```python
from build123d import *

# Parameters (mm, degrees)
EXTRUDE_2_DEPTH     = 10
SKETCH_2_R          = 10
CUT_EXTRUDE_1_DEPTH = 10
SKETCH_3_R          = 10
CUT_EXTRUDE_2_DEPTH = 10


with BuildPart() as part:
    # Эскиз1 → Бобышка-Вытянуть2 (new body)
    with BuildSketch(Plane.XY):
        with BuildLine():
            Line((0, 0), (-500, 0))
            ThreePointArc((-500, 0), (-515, 15), (-500, 30))
            Line((-500, 30), (0, 30))
            ThreePointArc((0, 30), (15, 15), (0, 0))
        make_face()
    extrude(amount=EXTRUDE_2_DEPTH)

    # Эскиз2 → Вырез-Вытянуть1 (cut)
    with BuildSketch(Plane(origin=(0, 0, 0), x_dir=(-1, 0, 0), z_dir=(0, 0, -1))):
        with Locations((0, 15)):
            Circle(SKETCH_2_R)
        with Locations((500, 15)):
            Circle(SKETCH_2_R)
    extrude(amount=-CUT_EXTRUDE_1_DEPTH, mode=Mode.SUBTRACT)

    # Эскиз3 → Вырез-Вытянуть2 (cut)
    with BuildSketch(Plane.XY.offset(10)):
        with Locations((-100, 15)):
            Circle(SKETCH_3_R)
    extrude(amount=-CUT_EXTRUDE_2_DEPTH, mode=Mode.SUBTRACT)


solid = part.part
```
Work out the finished part from the listing and answer in its coordinate system (mm). Give positions to 0.01 mm unless a question says otherwise; leave off trailing zeros. Write each loop counter-clockwise with the first axis right and the second up, starting at its lowest first coordinate (ties: lowest second). Pieces come first, ordered by that corner, then holes. Notation, with made-up numbers: (32.25, -2.5) -> (85.25, -2.5) arc R14 cw to (85.25, 19.5) -> close; hole circle Ø7 at (63.25, -13.5). An arc over 180 degrees is marked (long way). Write item = value, one per line.
Q1. For a pull along X with two mould halves and no side action, classify faces 1 (the cylindrical face through (-110, 15, 5)), 2 (the cylindrical face through (15, 15, 5)), 3 (the flat face through (-247, 0, 5)) as pulls with the +X half, pulls with the -X half, needs draft (parallel to the pull), parting line crosses it, or undercut.
Computed values:
face_1 = undercut
face_2 = pulls with the +X half
face_3 = needs draft
Q2. Consider line 1 along X through (y, z) = (14.25, 9.25); line 2 along Y through (x, z) = (-100, 3.75); line 3 along X through (y, z) = (20.75, 4). Determine where each line is inside the solid, lowest interval first.
Computed values:
line_1 = -514.98 to -509.97, -490.03 to -109.97, -90.03 to -9.97, 9.97 to 14.98
line_2 = 0 to 5, 25 to 30
line_3 = -513.85 to -508.18, -491.82 to -108.18, -91.82 to -8.18, 8.18 to 13.85
Q3. A flat-ended cylindrical pin translates along its axis: pin 1 Ø2 at (y, z) = (20, 6.5) entering from +X. Find the tip coordinate at first contact, or state that the pin passes through.
Computed values:
pin_1 = 14.46
Q4. Section A-A on z = 6.75 is taken. Determine the outline of the cut face in (x, y).
Computed values:
outline = (-500, 0) -> (0, 0) arc R15 ccw to (0, 30) -> (-500, 30) arc R15 ccw to start; hole circle Ø20 at (-500, 15); hole circle Ø20 at (-100, 15); hole circle Ø20 at (0, 15)
Q5. Section C-C on x = -100 is taken. Determine the outline of the cut face in (y, z), and give its area (3 significant figures).
Computed values:
outline = (0, 0) -> (5, 0) -> (5, 10) -> (0, 10) -> close; (25, 0) -> (30, 0) -> (30, 10) -> (25, 10) -> close
area = 100 mm^2
Q6. Section B-B on y = 15 is taken. Determine the outline of the cut face in (x, z), and give its area (3 significant figures).
Computed values:
outline = (-515, 0) -> (-510, 0) -> (-510, 10) -> (-515, 10) -> close; (-490, 0) -> (-110, 0) -> (-110, 10) -> (-490, 10) -> close; (-90, 0) -> (-10, 0) -> (-10, 10) -> (-90, 10) -> close; (10, 0) -> (15, 0) -> (15, 10) -> (10, 10) -> close
area = 4,700 mm^2
